```python
from build123d import *

# Parameters (mm, degrees)
SKETCH1_W           = 40
SKETCH1_H           = 40
BOSS_EXTRUDE1_DEPTH = 40
SKETCH2_W           = 10
SKETCH2_H           = 20
CUT_EXTRUDE1_DEPTH  = 40
SKETCH3_W           = 20
SKETCH3_H           = 20
CUT_EXTRUDE2_DEPTH  = 40
CUT_EXTRUDE3_DEPTH  = 40
SKETCH5_W           = 20
SKETCH5_H           = 20
CUT_EXTRUDE4_DEPTH  = 10
CUT_EXTRUDE6_DEPTH  = 43


with BuildPart() as part:
    # Sketch1 → Boss-Extrude1 (new body)
    with BuildSketch(Plane.XY):
        with Locations((20, 20)):
            Rectangle(SKETCH1_W, SKETCH1_H)
    extrude(amount=BOSS_EXTRUDE1_DEPTH)

    # Sketch2 → Cut-Extrude1 (cut)
    with BuildSketch(Plane.XY.offset(40)):
        with Locations((5, 30)):
            Rectangle(SKETCH2_W, SKETCH2_H)
        with Locations((35, 10)):
            Rectangle(SKETCH2_W, SKETCH2_H)
    extrude(amount=-CUT_EXTRUDE1_DEPTH, mode=Mode.SUBTRACT)

    # Sketch3 → Cut-Extrude2 (cut)
    with BuildSketch(Plane.ZY.offset(-10)):
        with Locations((30, 30)):
            Rectangle(SKETCH3_W, SKETCH3_H)
    extrude(amount=-CUT_EXTRUDE2_DEPTH, mode=Mode.SUBTRACT)

    # Sketch4 → Cut-Extrude3 (cut)
    with BuildSketch(Plane.ZY.offset(-10)):
        with BuildLine():
            Line((20, 40), (0, 40))
            Line((0, 40), (0, 20))
            ThreePointArc((0, 20), (5.857864376, 34.142135624), (20, 40))
        make_face()
    extrude(amount=-CUT_EXTRUDE3_DEPTH, mode=Mode.SUBTRACT)

    # Sketch5 → Cut-Extrude4 (cut)
    with BuildSketch(Plane(origin=(30, 0, 0), x_dir=(0, 0, -1), z_dir=(1, 0, 0))):
        with Locations((-30, 10)):
            Rectangle(SKETCH5_W, SKETCH5_H)
    extrude(amount=-CUT_EXTRUDE4_DEPTH, mode=Mode.SUBTRACT)

    # Sketch6 → Cut-Extrude6 (cut)
    with BuildSketch(Plane.ZY):
        with BuildLine():
            ThreePointArc((20, 0), (5.857864376, 5.857864376), (0, 20))
            Line((0, 20), (0, 0))
            Line((0, 0), (20, 0))
        make_face()
        with BuildLine():
            ThreePointArc((40, 20), (34.142135624, 5.857864376), (20, 0))
            Line((20, 0), (40, 0))
            Line((40, 0), (40, 20))
        make_face()
    extrude(amount=-CUT_EXTRUDE6_DEPTH, mode=Mode.SUBTRACT)


solid = part.part
```
Source: CAD feature listing. Evaluate the final solid. Frame: model axes, mm. A direction names the side the tool comes from. Round coordinates to 2 decimals unless told otherwise and drop trailing zeros. Loops run counter-clockwise (first coordinate to the right, second up) from the corner with the lowest first, then second, coordinate; pieces in that order, holes last. Notation, with made-up numbers: M 20.25,57 L 24.25,57 A29 ccw 24.25,78 Z; hole C 85,-12.75 d7. An arc over 180 degrees is marked long. Use a Markdown table: item, result. Add a question column.
1. Section query A-A on z = 7. Return the cut outline in (x, y).
2. Contact query for flat-ended pins moving along their axis: P1, Ø6, axis at x = 14.5, z = 10.5, coming from the +Y side; P2, Ø12, axis at x = 17.5, y = 13, coming from the -Z side (3 decimals); P3, Ø6, axis at x = 5, z = 6.5, coming from the -Y side; P4, Ø12, axis at x = 29.5, z = 35, coming from the -Y side. Output: stop coordinate, or through.
3. Section query C-C on y = 15.5. Return the cut outline in (x, z), then the cut area to 3 significant figures.
4. Section query D-D on z = 11. Return the cut outline in (x, y).
5. Reachability of faces 1 (the flat face through (20, 12, 28)), 2 (the flat face through (35, 20, 10)), 3 (the flat face through (0, 12, 20)), 4 (the flat face through (10, 28, 12)), 5 (the flat face through (40, 28, 12)) from +Z, -Z, +X, -X, +Y, -Y: full face, straight path, thin tool, end or side. Return the list, or none.
6. Line query: line 1 (X direction, y = 4, z = 12); line 2 (X direction, y = 26, z = 11.5); line 3 (Y direction, x = 17.5, z = 18.5). Output: solid intervals per line, ascending.
7. Section query B-B on x = 17.5. Return the cut outline in (y, z).
Reported:
| question | item | result |
|---|---|---|
| 1 | outline | M 0,4.8 L 30,4.8 L 30,20 L 40,20 L 40,35.2 L 10,35.2 L 10,20 L 0,20 Z |
| 2 | P1 | stops at y = 38.91 |
| 2 | P2 | stops at z = 0.025 |
| 2 | P3 | stops at y = 2.98 |
| 2 | P4 | passes through |
| 3 | outline | M 0,0.51 L 30,0.51 L 30,20 L 20,20 L 20,39.49 L 0,39.49 Z |
| 3 | area | 974 mm² |
| 4 | outline | M 0,2.14 L 30,2.14 L 30,20 L 40,20 L 40,37.86 L 10,37.86 L 10,20 L 0,20 Z |
| 5 | face 1 | +Z, +X, +Y, -Y |
| 5 | face 2 | +Z, -Z, +X, -Y |
| 5 | face 3 | +Z, -Z, -X, +Y, -Y |
| 5 | face 4 | +Z, -Z, -X, +Y |
| 5 | face 5 | +Z, -Z, +X, +Y, -Y |
| 6 | line 1 | x = 0 to 30 |
| 6 | line 2 | x = 10 to 40 |
| 6 | line 3 | y = 0.06 to 39.94 |
| 7 | outline | M 20,20 L 20,40 A20 ccw long 40,20 Z |
